Here's how the part is built. I have some questions about the finished solid (model axes, mm). A direction names the side the tool comes from. Round coordinates to 2 decimals unless told otherwise and drop trailing zeros. Write each loop counter-clockwise with the first axis right and the second up, starting at its lowest first coordinate (ties: lowest second). Pieces come first, ordered by that corner, then holes. Notation, with made-up numbers: (14, -18.5) -> (30, -18.5) arc R36 ccw to (30, 17.5) -> close; hole circle Ø8 at (60.5, -6). An arc over 180 degrees is marked (long way). Put each result on its own line as item: value. Start each with the question number.
1) If I drill on line 1 along X through (y, z) = (0.25, 10.5); line 2 along Y through (x, z) = (-6.55, 13.25) (3 decimals); line 3 along X through (y, z) = (3.25, 19.5), over which ranges is the centre line in solid material (lowest first)? Write a range as [from, to].
2) I want a section at C-C, the plane y = 1.25. List the corners of the cut face in (x, z) for me, then the cut area to 3 significant figures.
3) Will this pin go through, and if not, where does the flat tip stop? P1, Ø4, axis at y = 0, z = 22, coming from the +X side.
4) I want a section at B-B, the plane x = -6.6. List the corners of the cut face in (y, z) for me (3 decimals), then the cut area to 3 significant figures.
5) We'd pull the mould along X, two halves only. Please class faces 4 (the cylindrical face through (-6.58, 1.22, 12.32)), 5 (the flat face through (-7.227, 0, 12)), 6 (the flat face through (-6.4, 3.125, 12.3)): released by +X, released by -X, zero draft, split by the parting line, or undercut.
6) I want a section at A-A, the plane z = 20.5. List the corners of the cut face in (x, y) for me (3 decimals), then the cut area to 3 significant figures.
7) Which directions (+Z, -Z, +X, -X, +Y, -Y) give clear straight access to the entire face, cutting with the end or side of a thin tool? Please do faces 1 (the cylindrical face through (-6.595, -1.191, 12.325)), 2 (the flat face through (-7, 0, 0)), 3 (the flat face through (-6.4, -3.125, 12.3)).
from build123d import *

# Parameters (mm, degrees)
F1_DEPTH    = 25
F2_T1_DEPTH = 25


# Not quite as in the source:
# - a fillet or chamfer that OpenCascade refuses, or shapes differently, is made with other operations: its cross-section is extruded or revolved along the edge and cut away or added


with BuildPart() as f1:
    # F0 (on Top) → F1 (new body)
    with BuildSketch(Plane.XY):
        Polygon((-6.8274033331, 3.5), (-7.2274033331, 3.5), (-7.2274033331, 0), (-7.2274033331, -3.5), (-6.8274033331, -3.5), (-6.8274033331, -3.125), (-5.9274033331, -3.125), (-5.6274033331, -3.425), (-5.3675957119, -3.275), (-5.3675957119, -2.4848076211), (-5.9274033331, -1.925), (-6.8274033331, -1.925), (-6.8274033331, -0.6), (-6.8274033331, 0.6), (-6.8274033331, 1.925), (-5.9274033331, 1.925), (-5.3675957119, 2.4848076211), (-5.3675957119, 3.275), (-5.6274033331, 3.425), (-5.9274033331, 3.125), (-6.8274033331, 3.125), align=None)
    extrude(amount=F1_DEPTH)

    # F2: fillet of radius 2 on 2 edges, made by hand

    # F2_s2 → F2_t1 (join)
    with BuildSketch(Plane.XY):
        with BuildLine():
            ThreePointArc((-5.9274033331, 1.925), (-6.5880850192, 1.2033539892), (-6.8274033331, 0.2546706911))
            Line((-6.8274033331, 0.2546706911), (-6.8274033331, 1.925))
            Line((-6.8274033331, 1.925), (-5.9274033331, 1.925))
        make_face()
        with BuildLine():
            ThreePointArc((-6.8274033331, -0.2546706911), (-6.5880850192, -1.2033539892), (-5.9274033331, -1.925))
            Line((-5.9274033331, -1.925), (-6.8274033331, -1.925))
            Line((-6.8274033331, -1.925), (-6.8274033331, -0.2546706911))
        make_face()
    extrude(amount=F2_T1_DEPTH)


solid = f1.part
Findings:
1. line 1: x = [-7.23, -6.83]
1. line 2: y = [-3.125, -1.271], [1.271, 3.125]
1. line 3: x = [-7.23, -6.83], [-5.8, -5.37]
2. outline: (-7.23, 0) -> (-6.56, 0) -> (-6.56, 25) -> (-7.23, 25) -> close
2. area: 16.6 mm2
3. P1: stops at x = -5.85
4. outline: (-3.125, 0) -> (-1.181, 0) -> (-1.181, 25) -> (-3.125, 25) -> close; (1.181, 0) -> (3.125, 0) -> (3.125, 25) -> (1.181, 25) -> close
4. area: 97.2 mm2
5. face 4: released by +X
5. face 5: released by -X
5. face 6: undercut
6. outline: (-7.227, -3.5) -> (-6.827, -3.5) -> (-6.827, -3.125) -> (-5.927, -3.125) -> (-5.627, -3.425) -> (-5.368, -3.275) -> (-5.368, -2.485) -> (-5.927, -1.925) arc R2 cw to (-6.827, -0.255) -> (-6.827, 0.255) arc R2 cw to (-5.927, 1.925) -> (-5.368, 2.485) -> (-5.368, 3.275) -> (-5.627, 3.425) -> (-5.927, 3.125) -> (-6.827, 3.125) -> (-6.827, 3.5) -> (-7.227, 3.5) -> close
6. area: 7.09 mm2
7. face 1: +Z, -Z, +X
7. face 2: -Z, +X, -X, +Y, -Y
7. face 3: +Z, -Z, -Y
